For this review, take the finished solid that the model builds, in its own axes (mm). A direction names the side the tool comes from. Coordinates: 2 decimals unless noted, no trailing zeros. Write each loop counter-clockwise with the first axis right and the second up, starting at its lowest first coordinate (ties: lowest second). Pieces come first, ordered by that corner, then holes. Notation, with made-up numbers: M 8.5,-13.5 L 44.5,-13.5 A27 cw 44.5,19.5 Z; hole C -24,1.5 d3. An arc over 180 degrees is marked long. One line per question, with ' | ' between items.
from build123d import *

# Parameters (mm, degrees)
SKETCH_1_R                   = 25
EXTRUDE_1_DEPTH              = 5
SKETCH_2_R                   = 1
CUT_EXTRUDE_1_DEPTH          = 4
HOLE_WIZARD_M3_1_D           = 3.4
HOLE_WIZARD_M3_1_DEPTH       = 7.5
HOLE_WIZARD_M3_1_CSINK_D     = 6.6
HOLE_WIZARD_M3_1_CSINK_ANGLE = 90
HOLE_WIZARD_M3_1_TIP         = 1.021463052
SKETCH_4_R                   = 2
CUT_EXTRUDE_2_DEPTH          = 4
HOLE_WIZARD_M5_1_D           = 4.2
HOLE_WIZARD_M5_1_DEPTH       = 12.4
HOLE_WIZARD_M5_1_TIP         = 1.2618073
SKETCH_7_W                   = 78.33195998
SKETCH_7_H                   = 10
CUT_EXTRUDE_3_DEPTH          = 6
FILLET_1_R                   = 10
SKETCH_9_R                   = 6
CUT_EXTRUDE_5_DEPTH          = 10
SKETCH_10_W                  = 10
SKETCH_10_H                  = 11.68337521
CUT_EXTRUDE_6_DEPTH          = 10
FILLET_2_R                   = 1


with BuildPart() as part:
    # 草图1 → 凸台-拉伸1 (new body)
    with BuildSketch(Plane(origin=(0, 0, 0), x_dir=(1, 0, 0), z_dir=(0, 1, 0))):
        Circle(SKETCH_1_R)
    extrude(amount=EXTRUDE_1_DEPTH)

    # 草图2 → 切除-拉伸1 (cut)
    with BuildSketch(Plane(origin=(0, 5, 0), x_dir=(1, 0, 0), z_dir=(0, 1, 0))):
        with Locations((11.691342951, 6.75)):
            Circle(SKETCH_2_R)
        with Locations((11.691342951, -6.75)):
            Circle(SKETCH_2_R)
        with Locations((-11.691342951, -6.75)):
            Circle(SKETCH_2_R)
        with Locations((-11.691342951, 6.75)):
            Circle(SKETCH_2_R)
    extrude(amount=-CUT_EXTRUDE_1_DEPTH, mode=Mode.SUBTRACT)

    # M3 十字槽沉头木螺钉的锥形沉头孔1
    with Locations(Plane(origin=(11.691342951, 5, -6.75), x_dir=(0, 0, 1), z_dir=(0, 1, 0))):
        with Locations((0, 0), (13.5, 0), (13.5, -23.382685902), (0, -23.382685902)):
            CounterSinkHole(HOLE_WIZARD_M3_1_D / 2, HOLE_WIZARD_M3_1_CSINK_D / 2, depth=HOLE_WIZARD_M3_1_DEPTH, counter_sink_angle=HOLE_WIZARD_M3_1_CSINK_ANGLE)
            with Locations((0, 0, -(HOLE_WIZARD_M3_1_DEPTH + HOLE_WIZARD_M3_1_TIP / 2))):  # 118° drill point
                Cone(0, HOLE_WIZARD_M3_1_D / 2, HOLE_WIZARD_M3_1_TIP, mode=Mode.SUBTRACT)

    # 草图4 → 切除-拉伸2 (cut)
    with BuildSketch(Plane(origin=(0, 5, 0), x_dir=(1, 0, 0), z_dir=(0, 1, 0))):
        with Locations((-20, 0)):
            Circle(SKETCH_4_R)
        with Locations((20, 0)):
            Circle(SKETCH_4_R)
    extrude(amount=-CUT_EXTRUDE_2_DEPTH, mode=Mode.SUBTRACT)

    # M5 螺纹孔1
    with Locations(Plane(origin=(-20, 5, 0), x_dir=(0, 0, 1), z_dir=(0, 1, 0))):
        with Locations((0, 0), (0, 40)):
            Hole(HOLE_WIZARD_M5_1_D / 2, depth=HOLE_WIZARD_M5_1_DEPTH)
            with Locations((0, 0, -(HOLE_WIZARD_M5_1_DEPTH + HOLE_WIZARD_M5_1_TIP / 2))):  # 118° drill point
                Cone(0, HOLE_WIZARD_M5_1_D / 2, HOLE_WIZARD_M5_1_TIP, mode=Mode.SUBTRACT)

    # 草图7 → 切除-拉伸3 (cut, through all)
    with BuildSketch(Plane(origin=(0, 5, 0), x_dir=(1, 0, 0), z_dir=(0, 1, 0))):
        with Locations((0, 20)):
            Rectangle(SKETCH_7_W, SKETCH_7_H)
        with Locations((0, -20)):
            Rectangle(SKETCH_7_W, SKETCH_7_H)
    extrude(amount=-CUT_EXTRUDE_3_DEPTH, mode=Mode.SUBTRACT)

    # 圆角1
    fillet_1_edges = [part.edges().sort_by_distance(p)[0] for p in [
        (20, 2.5, 15),
        (-20, 2.5, 15),
        (-20, 2.5, -15),
        (20, 2.5, -15),
    ]]
    fillet(fillet_1_edges, radius=FILLET_1_R)

    # 草图9 → 切除-拉伸5 (cut)
    with BuildSketch(Plane(origin=(0, 5, 0), x_dir=(1, 0, 0), z_dir=(0, 1, 0))):
        Circle(SKETCH_9_R)
    extrude(amount=-CUT_EXTRUDE_5_DEPTH, mode=Mode.SUBTRACT)

    # 草图10 → 切除-拉伸6 (cut)
    with BuildSketch(Plane(origin=(0, 5, 0), x_dir=(1, 0, 0), z_dir=(0, 1, 0))):
        with Locations((0, 9.158312395)):
            Rectangle(SKETCH_10_W, SKETCH_10_H)
    extrude(amount=-CUT_EXTRUDE_6_DEPTH, mode=Mode.SUBTRACT)

    # 圆角2
    fillet_2_edges = [part.edges().sort_by_distance(p)[0] for p in [
        (-5, 2.5, -3.31662479),
        (5, 2.5, -3.31662479),
        (-5, 2.5, -15),
        (5, 2.5, -15),
    ]]
    fillet(fillet_2_edges, radius=FILLET_2_R)


solid = part.part
1) We need section D-D on y = 0.5. State the section outline as (x, z) points.
Responses:
outline: M -23.57,-8.33 A10 ccw -14.14,-15 L -6,-15 A1 ccw -5,-14 L -5,-3.61 A1 ccw -5.14,-3.09 A6 cw long 5.14,-3.09 A1 ccw 5,-3.61 L 5,-14 A1 ccw 6,-15 L 14.14,-15 A10 ccw 23.57,-8.33 A25 ccw 23.57,8.33 A10 ccw 14.14,15 L -14.14,15 A10 ccw -23.57,8.33 A25 ccw Z; hole C -20,0 d4.2; hole C -11.69,-6.75 d3.4; hole C -11.69,6.75 d3.4; hole C 11.69,-6.75 d3.4; hole C 11.69,6.75 d3.4; hole C 20,0 d4.2
2) The part is to be moulded in two halves that separate along X. For faces 1 (the flat face through (10, 3, -15)), 2 (the cylindrical face through (10.032, 1.676, -6.381)), 3 (the cylindrical face through (-19.99, 2.46, 13.11)), say which applies: +X half, -X half, draft (parallel to the pull), parting line (faces both ways), or undercut.
Responses:
face 1: draft | face 2: undercut | face 3: -X half
3) Insertion check: pin 1 Ø4 at (x, z) = (-11.69, 6.75) entering from -Y; pin 2 Ø1.5 at (y, z) = (3.5, 0) entering from +X; pin 3 Ø1 at (y, z) = (1.5, 3) entering from +X; pin 4 Ø2.5 at (y, z) = (1.5, -7) entering from +X. Each pin has a flat end and moves straight along its axis. Give the tip position at first contact, or say it passes through.
Responses:
pin 1: y = 0 | pin 2: x = 25 | pin 3: x = 24.87 | pin 4: x = 24.33
4) We need section B-B on z = -12.75. State the section outline as (x, y) points.
Responses:
outline: M -20.46,0 L -5,0 L -5,5 L -20.46,5 Z; M 5,0 L 20.46,0 L 20.46,5 L 5,5 Z
5) Machinability: for faces 4 (the cylindrical face through (-5.301, 2.465, -14.715)), 5 (the flat face through (0, 3, 15)), which of the approach directions +Z, -Z, +X, -X, +Y, -Y give a long, thin tool a straight path to every point of the face, cutting with its end or side? Answer none if there is none.
Responses:
face 4: -Z, +Y, -Y | face 5: +Z, +X, -X, +Y, -Y
6) To check wall thickness, follow line 1 along X through (y, z) = (3.75, 0); line 2 along X through (y, z) = (3.25, -6.75); line 3 along Z through (x, y) = (-12.5, 0.3). State the ranges of each line that lie inside material, in increasing order. Write a range as [from, to].
Responses:
line 1: [-25, -22.1], [-17.9, -6], [6, 17.9], [22.1, 25] | line 2: [-24.07, -13.39], [-9.99, -5], [5, 9.99], [13.39, 24.07] | line 3: [-15, -8.25], [-5.25, 5.25], [8.25, 15]
7) We need section C-C on x = -20. State the section outline as (y, z) points.
Responses:
outline: M 0,-13.1 L 5,-13.1 L 5,-2.1 L 0,-2.1 Z; M 0,2.1 L 5,2.1 L 5,13.1 L 0,13.1 Z
8) We need section A-A on z = 0. State the section outline as (x, y) points, then the cut area to 3 significant figures.
Responses:
outline: M -25,0 L -22.1,0 L -22.1,5 L -25,5 Z; M -17.9,0 L -6,0 L -6,5 L -17.9,5 Z; M 6,0 L 17.9,0 L 17.9,5 L 6,5 Z; M 22.1,0 L 25,0 L 25,5 L 22.1,5 Z | area: 148 mm^2
